from build123d import *

# Parameters (mm, degrees)
SKETCH2_R          = 6
CUT_EXTRUDE1_DEPTH = 26.88


with BuildPart() as part:
    # Sketch1 → Revolve1 (revolve)
    with BuildSketch(Plane.XY.offset(40)):
        Polygon((5.353553391, 0), (17.146446609, 0), (17.5, 0.353553391), (17.5, 10), (19.995, 10), (26.855, 16.86), (16.085548044, 25.88), (12.205548044, 22), (5, 22), (5, 0.353553391), align=None)
    revolve(axis=Axis((0, 25.88, 40), (0, -1, 0)))

    # Sketch2 → Cut-Extrude1 (cut, through all)
    with BuildSketch(Plane.XZ):
        with Locations((0, 40)):
            Circle(SKETCH2_R)
    extrude(amount=-CUT_EXTRUDE1_DEPTH, mode=Mode.SUBTRACT)


solid = part.part
Source: CAD feature listing. Evaluate the final solid. Frame: model axes, mm. A direction names the side the tool comes from. Coordinates: 2 decimals unless noted, no trailing zeros. Loops run counter-clockwise (first coordinate to the right, second up) from the corner with the lowest first, then second, coordinate; pieces in that order, holes last. Notation, with made-up numbers: (21.25, 28) -> (40.25, 28) arc R12 ccw to (40.25, 35) -> close; hole circle Ø6 at (33, 72.5). An arc over 180 degrees is marked (long way). Answer in a Markdown table with one row per item. Add a question column.
Q1. Contact query for flat-ended pins moving along their axis: pin 1 Ø2 at (y, z) = (18.5, 25) entering from -X; pin 2 Ø1.5 at (x, z) = (5, 30) entering from +Y; pin 3 Ø12 at (x, y) = (-14, 9) entering from -Z. Output: stop coordinate, or through.
Q2. Section D-D on y = 14. Return the cut outline in (x, z) (3 decimals), and give its area (3 significant figures).
Q3. Section C-C on y = 3.75. Return the cut outline in (x, z).
Q4. Ray query, line 1 along Z through (x, y) = (0, 9); line 2 along Y through (x, z) = (-5.5, 37.5); line 3 along Z through (x, y) = (0, 17). Return the intervals inside material, ascending.
Q5. Section A-A on z = 40. Return the cut outline in (x, y) (3 decimals).
Q6. Pull-direction query (X, two-part tool) for faces 3 (the face through (-2.16, 25.44, 56.47)), 4 (the face through (-6, 22, 37)), 5 (the face through (0, 10, 22)); classes: pulls with the +X half, pulls with the -X half, needs draft (parallel to the pull), parting line crosses it, or undercut.
Q7. Section B-B on x = 0. Return the cut outline in (y, z) (3 decimals), and give its area (3 significant figures).
Q8. Reachability of faces 1 (the face through (-1.301, 10.846, 34.143)), 2 (the face through (-2.28, 5.24, 57.35)) from +Z, -Z, +X, -X, +Y, -Y: full face, straight path, thin tool, end or side. Return the list, or none.
Computed values:
| question | item | result |
|---|---|---|
| 1 | pin 1 | stops at x = -21.5 |
| 1 | pin 2 | stops at y = 22 |
| 1 | pin 3 | stops at z = 18.42 |
| 2 | outline | circle Ø47.99 at (0, 40); hole circle Ø12 at (0, 40) |
| 2 | area | 1,700 mm^2 |
| 3 | outline | circle Ø35 at (0, 40); hole circle Ø12 at (0, 40) |
| 4 | line 1 | z = 22.5 to 34, 46 to 57.5 |
| 4 | line 2 | y = 0 to 22 |
| 4 | line 3 | z = 13.31 to 34, 46 to 66.69 |
| 5 | outline | (-26.855, 16.86) -> (-19.995, 10) -> (-17.5, 10) -> (-17.5, 0.354) -> (-17.146, 0) -> (-6, 0) -> (-6, 22) -> (-12.206, 22) -> (-16.086, 25.88) -> close; (6, 0) -> (17.146, 0) -> (17.5, 0.354) -> (17.5, 10) -> (19.995, 10) -> (26.855, 16.86) -> (16.086, 25.88) -> (12.206, 22) -> (6, 22) -> close |
| 6 | face 3 | parting line crosses it |
| 6 | face 4 | undercut |
| 6 | face 5 | needs draft |
| 7 | outline | (0, 22.854) -> (0.354, 22.5) -> (10, 22.5) -> (10, 20.005) -> (16.86, 13.145) -> (25.88, 23.914) -> (22, 27.794) -> (22, 34) -> (0, 34) -> close; (0, 46) -> (22, 46) -> (22, 52.206) -> (25.88, 56.086) -> (16.86, 66.855) -> (10, 59.995) -> (10, 57.5) -> (0.354, 57.5) -> (0, 57.146) -> close |
| 7 | area | 685 mm^2 |
| 8 | face 1 | +Y, -Y |
| 8 | face 2 | -Y |
